Part model, mm, in its own coordinate system. A direction names the side the tool comes from. Give positions to 0.01 mm unless a question says otherwise; leave off trailing zeros. Order: outer loops, then holes, each group sorted by start corner. A loop starts at its lowest first (then second) coordinate and runs counter-clockwise, first axis right, second up.
1. Probe line 1 (Y direction, x = -14, z = 17.25); line 2 (Y direction, x = -33, z = 11.5); line 3 (X direction, y = -3, z = 11.75). List the from-to ranges inside material, lowest first.
2. Slice it at A-A on x = -24. List the corners of the cut face in (y, z), and give its area (3 significant figures).
3. Which spindle directions (+Z, -Z, +X, -X, +Y, -Y) get a long thin tool onto all of the face, cutting with end or side? Do faces 4 (the flat face through (-29, 22, 1)), 5 (the flat face through (25, -20, 0)), 6 (the flat face through (-12, 2, 12)). Say none if no direction does.
4. Mould opens along X. For faces 1 (the flat face through (44, 15, 12)), 2 (the flat face through (25, -20, 25)), 3 (the flat face through (16, 22, 1)) say: +X half, -X half, draft (parallel to the pull), parting line (faces both ways), or undercut.
5. Drop flat-ended pins along their axis: pin 1 Ø4 at (y, z) = (-80.5, 18.5) entering from -X; pin 2 Ø6 at (x, z) = (-9, 13) entering from -Y; pin 3 Ø3 at (y, z) = (14.5, 5) entering from +X; pin 4 Ø3 at (x, y) = (15.5, -50.5) entering from -Z. Give the stop position or say it passes through.
6. Slice it at B-B on y = -17. Give the number of separate pieces and of enclosed holes in the cut face, and give its area (3 significant figures).
from build123d import *

# Parameters (mm, degrees)
F0_W     = 42
F0_H     = 22
F0_W_2   = 6
F0_H_2   = 2
F1_DEPTH = 25
F2_W     = 30
F2_H     = 19
F2_W_2   = 20
F2_H_2   = 6.5
F2_W_3   = 12
F3_DEPTH = 22
F4_DEPTH = 55
F5_DEPTH = 34
F6_DEPTH = 27


with BuildPart() as f1:
    # F0 (on Top) → F1 (new body)
    with BuildSketch(Plane.XY):
        Polygon((44, 30), (-44, 30), (-44, -30), (6, -30), (44, -30), (44, 0), align=None)
        with Locations((-19, -15)):
            Rectangle(F0_W, F0_H, mode=Mode.SUBTRACT)
        with Locations((-29, 23)):
            Rectangle(F0_W_2, F0_H_2, mode=Mode.SUBTRACT)
        with Locations((-14, 23)):
            Rectangle(F0_W_2, F0_H_2, mode=Mode.SUBTRACT)
        with Locations((1, 23)):
            Rectangle(F0_W_2, F0_H_2, mode=Mode.SUBTRACT)
        with Locations((16, 23)):
            Rectangle(F0_W_2, F0_H_2, mode=Mode.SUBTRACT)
        with Locations((31, 23)):
            Rectangle(F0_W_2, F0_H_2, mode=Mode.SUBTRACT)
        with BuildLine():
            add(Edge.make_bspline(
                [(44, 0), (53.346686, -31.095194), (86.653314, -53.904806), (96, -85)],
                knots=[0, 0, 0, 0, 99.644368, 99.644368, 99.644368, 99.644368], degree=3))
            Line((44, 0), (44, -30))
            Line((44, -30), (6, -30))
            ThreePointArc((6, -30), (16.724801, -38.440392), (17.787344, -52.046735))
            Line((17.787344, -52.046735), (19.384056, -54.586521))
            ThreePointArc((19.384056, -54.586521), (28.940376, -64.33015), (28.252722, -77.960582))
            Line((28.252722, -77.960582), (29.849434, -80.500368))
            ThreePointArc((29.849434, -80.500368), (39.700482, -86.135868), (40.449604, -97.460214))
            Line((40.449604, -97.460214), (42.046316, -100))
            Line((42.046316, -100), (96, -85))
        make_face()
    extrude(amount=F1_DEPTH)

    # F2 (on face) → F3 (cut)
    with BuildSketch(Plane(origin=(0, 30, 0), x_dir=(-1, 0, 0), z_dir=(0, 1, 0))):
        with Locations((-26, 12.5)):
            Rectangle(F2_W, F2_H)
        Polygon((32, 22), (-11, 22), (-11, 3), (32, 3), (32, 9.25), (12, 9.25), (12, 15.75), (32, 15.75), align=None)
        with Locations((22, 12.5)):
            Rectangle(F2_W_2, F2_H_2)
        with Locations((38, 12.5)):
            Rectangle(F2_W_3, F2_H_2)
    extrude(amount=-F3_DEPTH, mode=Mode.SUBTRACT)

    # F2 (on face) → F4 (cut)
    with BuildSketch(Plane(origin=(0, 30, 0), x_dir=(-1, 0, 0), z_dir=(0, 1, 0))):
        with Locations((-26, 12.5)):
            Rectangle(F2_W, F2_H)
    extrude(amount=-F4_DEPTH, mode=Mode.SUBTRACT)

    # F2 (on face) → F5 (cut, through all)
    with BuildSketch(Plane(origin=(0, 30, 0), x_dir=(-1, 0, 0), z_dir=(0, 1, 0))):
        with Locations((22, 12.5)):
            Rectangle(F2_W_2, F2_H_2)
    extrude(amount=-F5_DEPTH, mode=Mode.SUBTRACT)

    # F2 (on face) → F6 (cut)
    with BuildSketch(Plane(origin=(0, 30, 0), x_dir=(-1, 0, 0), z_dir=(0, 1, 0))):
        with Locations((38, 12.5)):
            Rectangle(F2_W_3, F2_H_2)
    extrude(amount=-F6_DEPTH, mode=Mode.SUBTRACT)


solid = f1.part
Data:
1. line 1: y = -30 to -26, -4 to 8
1. line 2: y = -30 to -26, -4 to 3
1. line 3: x = -44 to -32, -12 to 11, 41 to 44.98
2. outline: (-30, 0) - (-26, 0) - (-26, 25) - (-30, 25) - close; (-4, 0) - (30, 0) - (30, 3) - (8, 3) - (8, 9.25) - (-4, 9.25) - close; (-4, 15.75) - (8, 15.75) - (8, 22) - (30, 22) - (30, 25) - (-4, 25) - close
2. area: 454 mm2
3. face 4: +Z, -Z
3. face 5: -Z, +X, -X, +Y, -Y
3. face 6: +Y
4. face 1: +X half
4. face 2: draft
4. face 3: undercut
5. pin 1: stops at x = 28.59
5. pin 2: stops at y = -30
5. pin 3: stops at x = 44
5. pin 4: passes through
6. separate pieces: 2
6. enclosed holes: 1
6. area: 771 mm2
